Source: three-view drawing plus pictorial views. Frame: mm from the lowest corner of the part. Round coordinates to 2 decimals unless told otherwise and drop trailing zeros. Write each loop counter-clockwise with the first axis right and the second up, starting at its lowest first coordinate (ties: lowest second). Pieces come first, ordered by that corner, then holes. Notation, with made-up numbers: M 11.25,56 L 40.25,56 A19 ccw 40.25,89 Z; hole C 82,40 d2. An arc over 180 degrees is marked long. Answer as CSV lines item,"result". Start each with the question number.
Q1. Section query A-A on y = 35. Output: boundary loops of the cut face in (x, z), and give its area (3 significant figures).
Q2. Ray query, probe 1 along Y at (x, z) = (35, 107.95); probe 2 along Z at (x, y) = (35, 68); probe 3 along Z at (x, y) = (41, 27.5). Return the intervals inside material, ascending.
Q3. Mould query, pull axis Y, two halves, no side actions, for the marked faces 1 and 2. Classes: pulls with the +Y half, pulls with the -Y half, needs draft (parallel to the pull), parting line crosses it, or undercut.
Q4. Section query C-C on z = 5. Output: boundary loops of the cut face in (x, y), and give its area (3 significant figures).
Q5. Section query D-D on y = 63. Output: boundary loops of the cut face in (x, z).
Q6. First-contact query: pin 1 (8 mm diameter, centred on x = 11, y = 32.5, fed in from -Z); pin 2 (1.8 mm diameter, centred on y = 35, z = 5, fed in from -X); pin 3 (12 mm diameter, centred on y = 22.5, z = 59.5, fed in from +X); pin 4 (2 mm diameter, centred on y = 10, z = 91.5, fed in from +X). Flat tips, straight axial feed; report the tip coordinate or a pass-through.
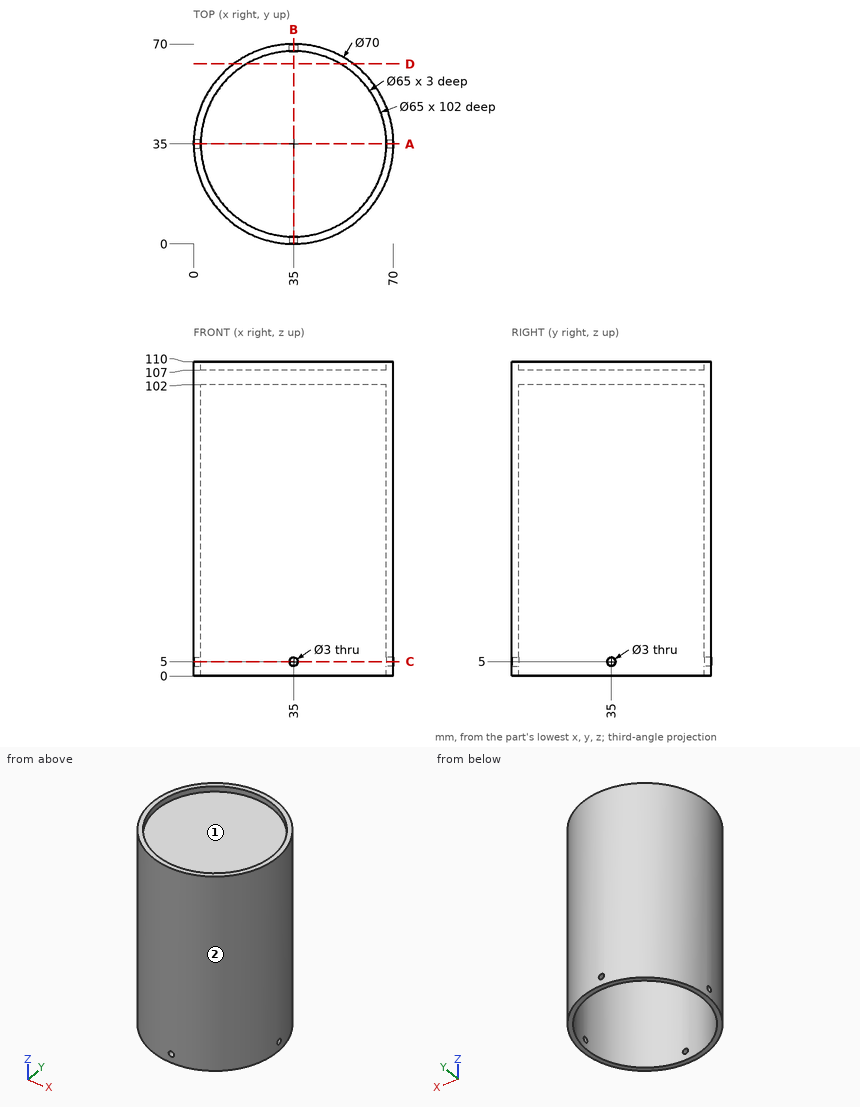
Entries:
1,outline,"M 0,0 L 2.5,0 L 2.5,3.5 L 0,3.5 Z; M 0,6.5 L 2.5,6.5 L 2.5,102 L 67.5,102 L 67.5,6.5 L 70,6.5 L 70,110 L 67.5,110 L 67.5,107 L 2.5,107 L 2.5,110 L 0,110 Z; M 67.5,0 L 70,0 L 70,3.5 L 67.5,3.5 Z"
1,area,"860 mm^2"
2,probe 1,"y = 0 to 2.5, 67.5 to 70"
2,probe 2,"z = 0 to 3.5, 6.5 to 110"
2,probe 3,"z = 102 to 107"
3,face 1,"undercut"
3,face 2,"parting line crosses it"
4,outline,"M 0.03,33.5 A35 ccw 33.5,0.03 L 33.5,2.53 A32.5 cw 2.53,33.5 Z; M 0.03,36.5 L 2.53,36.5 A32.5 cw 33.5,67.47 L 33.5,69.97 A35 ccw Z; M 36.5,0.03 A35 ccw 69.97,33.5 L 67.47,33.5 A32.5 cw 36.5,2.53 Z; M 36.5,67.47 A32.5 cw 67.47,36.5 L 69.97,36.5 A35 ccw 36.5,69.97 Z"
4,area,"500 mm^2"
5,outline,"M 14,0 L 18.5,0 L 18.5,102 L 51.5,102 L 51.5,0 L 56,0 L 56,110 L 51.5,110 L 51.5,107 L 18.5,107 L 18.5,110 L 14,110 Z"
6,pin 1,"stops at z = 102"
6,pin 2,"passes through"
6,pin 3,"stops at x = 69.39"
6,pin 4,"stops at x = 60.48"
